The model under review builds one solid part; all positions refer to its coordinate system, in mm. Face numbers are marked on the shaded views. A direction names the side the tool comes from. Round coordinates to 2 decimals unless told otherwise and drop trailing zeros. Order: outer loops, then holes, each group sorted by start corner. A loop starts at its lowest first (then second) coordinate and runs counter-clockwise, first axis right, second up.
1) To check wall thickness, follow L1, parallel to X at y = 2.15, z = 0; L2, parallel to X at y = 2.4, z = 5.75; L3, parallel to Z at x = -5.5, y = 2.9. State the ranges of each line that lie inside material, in increasing order.
2) Mouldability with a two-part tool opening along X and no side actions: class the marked faces 1, 2 and 3 as pulls with the +X half, pulls with the -X half, needs draft (parallel to the pull), parting line crosses it, or undercut.
3) Consider section C-C (z = 0). Give the boundary of the cut face in (x, y), then the cut area to 3 significant figures.
4) Consider section D-D (y = 2.3). Give the number of separate pieces and of enclosed holes in the cut face, then the cut area to 3 significant figures.
5) Clearance check with flat-ended pins moving along their axes: P1, Ø0.8, axis at y = 3, z = -1.5, coming from the -X side; P2, Ø0.8, axis at y = 2.5, z = 3, coming from the +X side; P3, Ø2, axis at x = -2, y = 3, coming from the -Z side. State where each tip first meets the part, or that it passes through.
6) Consider section A-A (y = 3.5). Give the boundary of the cut face in (x, z).
7) Machinability: for the marked faces 4, 5, 6, 7 and 8, which of the approach directions +Z, -Z, +X, -X, +Y, -Y give a long, thin tool a straight path to every point of the face, cutting with its end or side? Answer none if there is none.
8) Consider section B-B (x = 7.75). Give the boundary of the cut face in (y, z).
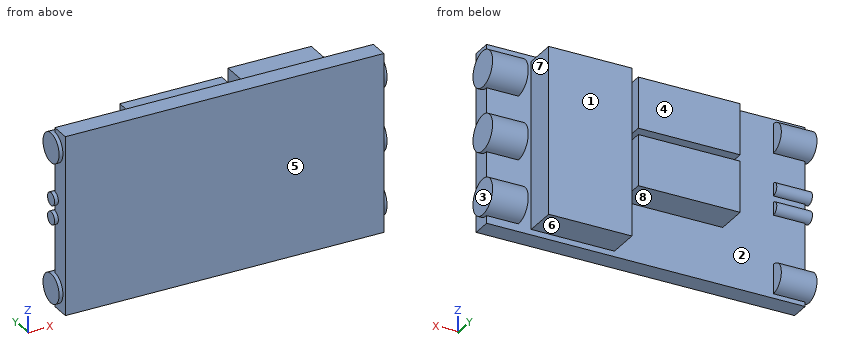
from build123d import *

# Parameters (mm, degrees)
SKIZZE1_W            = 25
SKIZZE1_H            = 14
PLATINE_DEPTH        = 1.5
SKIZZE2_W            = 6.530722005
SKIZZE2_H            = 13.138578522
MOSFETS_DEPTH        = 2.5
SKIZZE4_W            = 8
SKIZZE4_H            = 4
WEITERE_ICS_DEPTH    = 2.5
LOT_MOTOR_DEPTH      = 0.3
LOT_MOTOR_DEPTH_BACK = 2.5
SKIZZE5_R            = 1.4
LOT_PDB_DEPTH        = 0.3
LOT_PDB_DEPTH_BACK   = 2.5
SKIZZE6_R            = 1.15
LOT_FC_DEPTH         = 0.3
LOT_FC_DEPTH_BACK    = 2.5
SKIZZE7_R            = 0.5


with BuildPart() as part:
    # Skizze1 → Platine (new body)
    with BuildSketch(Plane(origin=(0, 0, 0), x_dir=(1, 0, 0), z_dir=(0, 1, 0))):
        Rectangle(SKIZZE1_W, SKIZZE1_H)
    extrude(amount=PLATINE_DEPTH)

    # Skizze2 → MOSFETs (add)
    with BuildSketch(Plane(origin=(0, 1.5, 0), x_dir=(1, 0, 0), z_dir=(0, 1, 0))):
        with Locations((5.733665382, 0)):
            Rectangle(SKIZZE2_W, SKIZZE2_H)
    extrude(amount=MOSFETS_DEPTH)

    # Skizze4 → Weitere_ICs (add)
    with BuildSketch(Plane(origin=(0, 1.5, 0), x_dir=(1, 0, 0), z_dir=(0, 1, 0))):
        with Locations((-2.03169562, -4)):
            Rectangle(SKIZZE4_W, SKIZZE4_H)
        with Locations((-2.03169562, 0.5)):
            Rectangle(SKIZZE4_W, SKIZZE4_H)
    extrude(amount=WEITERE_ICS_DEPTH)

    # Skizze5 → Lot_Motor (add, two sides: drawn at the far end of the back side and taken through both)
    with BuildSketch(Plane(origin=(12.5, 0, 0), x_dir=(0, 0, -1), z_dir=(1, 0, 0)).offset(-LOT_MOTOR_DEPTH_BACK)):
        with Locations((-5, 1.5)):
            Circle(SKIZZE5_R)
        with Locations((0, 1.5)):
            Circle(SKIZZE5_R)
        with Locations((5, 1.5)):
            Circle(SKIZZE5_R)
    extrude(amount=LOT_MOTOR_DEPTH + LOT_MOTOR_DEPTH_BACK)

    # Skizze6 → Lot_PDB (add, two sides: drawn at the far end of the back side and taken through both)
    with BuildSketch(Plane.ZY.offset(12.5).offset(-LOT_PDB_DEPTH_BACK)):
        with Locations((-5.5, 1.5)):
            Circle(SKIZZE6_R)
        with Locations((5.5, 1.5)):
            Circle(SKIZZE6_R)
    extrude(amount=LOT_PDB_DEPTH + LOT_PDB_DEPTH_BACK)

    # Skizze7 → Lot_FC (add, two sides: drawn at the far end of the back side and taken through both)
    with BuildSketch(Plane.ZY.offset(12.5).offset(-LOT_FC_DEPTH_BACK)):
        with Locations((1.5, 1.5)):
            Circle(SKIZZE7_R)
        with Locations((0, 1.5)):
            Circle(SKIZZE7_R)
    extrude(amount=LOT_FC_DEPTH + LOT_FC_DEPTH_BACK)


solid = part.part
Answer below:
1. L1: x = -6.03 to 1.97, 2.47 to 9, 10 to 12.8
1. L2: x = -12.8 to -10, -6.03 to 1.97, 2.47 to 9, 10 to 12.8
1. L3: z = -2.5 to 1.5, 2 to 6
2. face 1: needs draft
2. face 2: undercut
2. face 3: pulls with the +X half
3. outline: (-12.8, 1) - (-12.5, 1) - (-12.5, 0) - (12.5, 0) - (12.5, 0.1) - (12.8, 0.1) - (12.8, 2.9) - (10, 2.9) - (10, 1.5) - (9, 1.5) - (9, 4) - (2.47, 4) - (2.47, 1.5) - (1.97, 1.5) - (1.97, 4) - (-6.03, 4) - (-6.03, 1.5) - (-10, 1.5) - (-10, 2) - (-12.8, 2) - close
3. area: 79.7 mm2
4. separate pieces: 8
4. enclosed holes: 0
4. area: 178 mm2
5. P1: stops at x = -6.03
5. P2: stops at x = 9
5. P3: stops at z = -2.5
6. outline: (-6.03, -2.5) - (1.97, -2.5) - (1.97, 1.5) - (-6.03, 1.5) - close; (-6.03, 2) - (1.97, 2) - (1.97, 6) - (-6.03, 6) - close; (2.47, -6.57) - (9, -6.57) - (9, 6.57) - (2.47, 6.57) - close
7. face 4: +Z, -Z, +X, -X, +Y
7. face 5: +Z, -Z, +X, -X, -Y
7. face 6: -Z, +X, +Y
7. face 7: +Z, -Z, +Y
7. face 8: -Z, -X, +Y
8. outline: (0, -7) - (1.5, -7) - (1.5, -6.57) - (4, -6.57) - (4, 6.57) - (1.5, 6.57) - (1.5, 7) - (0, 7) - close
